```python
from build123d import *

# Parameters (mm, degrees)
F1_DEPTH  = 31.5
F2_R      = 3
F2_R_2    = 1.5
F3_DEPTH  = 5
F4_DEPTH  = 2
F2_R_3    = 4
F5_DEPTH  = 1
F6_DEPTH  = 4
F7_R      = 1.5
F8_DEPTH  = 31.5010001
F7_R_2    = 4
F9_DEPTH  = 2
F10_DEPTH = 33.501


with BuildPart() as f1:
    # F0 (on Top) → F1 (new body)
    with BuildSketch(Plane.XY):
        with BuildLine():
            Line((7.9372539332, -14.75), (0, -14.75))
            Line((0, -14.75), (0, -16.75))
            ThreePointArc((0, -16.75), (4.0926763859, -16.2423058708), (7.9372539332, -14.75))
        make_face()
        with BuildLine():
            ThreePointArc((16.75, 0), (16.2423058708, -4.0926763859), (14.75, -7.9372539332))
            Line((14.75, -7.9372539332), (14.75, -14.75))
            Line((14.75, -14.75), (7.9372539332, -14.75))
            ThreePointArc((7.9372539332, -14.75), (4.0926763859, -16.2423058708), (0, -16.75))
            Line((0, -16.75), (16.75, -16.75))
            Line((16.75, -16.75), (16.75, 0))
        make_face()
        with BuildLine():
            Line((14.75, -14.75), (14.75, -7.9372539332))
            ThreePointArc((14.75, -7.9372539332), (11.8440385849, -11.8440385849), (7.9372539332, -14.75))
            Line((7.9372539332, -14.75), (14.75, -14.75))
        make_face()
        with BuildLine():
            Line((14.75, -7.9372539332), (14.75, 0))
            ThreePointArc((14.75, 0), (10.4298250225, -10.4298250225), (0, -14.75))
            Line((0, -14.75), (7.9372539332, -14.75))
            ThreePointArc((7.9372539332, -14.75), (11.8440385849, -11.8440385849), (14.75, -7.9372539332))
        make_face()
        with BuildLine():
            ThreePointArc((0, -14.75), (10.4298250225, -10.4298250225), (14.75, 0))
            ThreePointArc((14.75, 0), (10.4298250225, 10.4298250225), (0, 14.75))
            Line((0, 14.75), (0, 12.75))
            ThreePointArc((0, 12.75), (9.0156114601, 9.0156114601), (12.75, 0))
            ThreePointArc((12.75, 0), (9.0156114601, -9.0156114601), (0, -12.75))
            Line((0, -12.75), (0, -14.75))
        make_face()
        with BuildLine():
            Line((14.75, 7.9372539332), (14.75, 0))
            Line((14.75, 0), (14.75, -7.9372539332))
            ThreePointArc((14.75, -7.9372539332), (16.2423058708, -4.0926763859), (16.75, 0))
            ThreePointArc((16.75, 0), (16.2423058708, 4.0926763859), (14.75, 7.9372539332))
        make_face()
        with BuildLine():
            ThreePointArc((0, 14.75), (10.4298250225, 10.4298250225), (14.75, 0))
            Line((14.75, 0), (14.75, 7.9372539332))
            ThreePointArc((14.75, 7.9372539332), (11.8440385849, 11.8440385849), (7.9372539332, 14.75))
            Line((7.9372539332, 14.75), (0, 14.75))
        make_face()
        with BuildLine():
            Line((14.75, 14.75), (14.75, 7.9372539332))
            ThreePointArc((14.75, 7.9372539332), (16.2423058708, 4.0926763859), (16.75, 0))
            Line((16.75, 0), (16.75, 16.75))
            Line((16.75, 16.75), (0, 16.75))
            ThreePointArc((0, 16.75), (4.0926763859, 16.2423058708), (7.9372539332, 14.75))
            Line((7.9372539332, 14.75), (14.75, 14.75))
        make_face()
        with BuildLine():
            ThreePointArc((7.9372539332, 14.75), (11.8440385849, 11.8440385849), (14.75, 7.9372539332))
            Line((14.75, 7.9372539332), (14.75, 14.75))
            Line((14.75, 14.75), (7.9372539332, 14.75))
        make_face()
        with BuildLine():
            Line((0, 16.75), (0, 14.75))
            Line((0, 14.75), (7.9372539332, 14.75))
            ThreePointArc((7.9372539332, 14.75), (4.0926763859, 16.2423058708), (0, 16.75))
        make_face()
        with BuildLine():
            Line((0, 12.75), (0, 14.75))
            ThreePointArc((0, 14.75), (-10.4298250296, 10.4298250154), (-14.75, -2e-08))
            ThreePointArc((-14.75, -2e-08), (-10.4298250154, -10.4298250296), (0, -14.75))
            Line((0, -14.75), (0, -12.75))
            ThreePointArc((0, -12.75), (-12.75, 0), (0, 12.75))
        make_face()
        with BuildLine():
            ThreePointArc((-14.75, -2e-08), (-10.4298250296, 10.4298250154), (0, 14.75))
            Line((0, 14.75), (-7.9372539332, 14.75))
            ThreePointArc((-7.9372539332, 14.75), (-11.8440385849, 11.8440385849), (-14.75, 7.9372539332))
            Line((-14.75, 7.9372539332), (-14.75, -2e-08))
        make_face()
        with BuildLine():
            Line((-7.9372539332, 14.75), (0, 14.75))
            Line((0, 14.75), (0, 16.75))
            ThreePointArc((0, 16.75), (-4.0926763859, 16.2423058708), (-7.9372539332, 14.75))
        make_face()
        with BuildLine():
            Line((-14.75, -7.9372539332), (-14.75, -2e-08))
            Line((-14.75, -2e-08), (-14.75, 7.9372539332))
            ThreePointArc((-14.75, 7.9372539332), (-16.2423058693, 4.092676392), (-16.75, 1.25e-08))
            ThreePointArc((-16.75, 1.25e-08), (-16.2423058723, -4.0926763799), (-14.75, -7.9372539332))
        make_face()
        with BuildLine():
            Line((-7.9372539332, -14.75), (0, -14.75))
            ThreePointArc((0, -14.75), (-10.4298250154, -10.4298250296), (-14.75, -2e-08))
            Line((-14.75, -2e-08), (-14.75, -7.9372539332))
            ThreePointArc((-14.75, -7.9372539332), (-11.8440385849, -11.8440385849), (-7.9372539332, -14.75))
        make_face()
        with BuildLine():
            Line((0, -16.75), (0, -14.75))
            Line((0, -14.75), (-7.9372539332, -14.75))
            ThreePointArc((-7.9372539332, -14.75), (-4.0926763859, -16.2423058708), (0, -16.75))
        make_face()
    extrude(amount=F1_DEPTH)

    # F2 (on face) → F3 (cut)
    with BuildSketch(Plane.YZ.offset(16.75)):
        with Locations((0, 24)):
            Circle(F2_R)
        with Locations((0, 24)):
            Circle(F2_R_2, mode=Mode.SUBTRACT)
        with Locations((0, 7.5)):
            Circle(F2_R)
        with Locations((0, 7.5)):
            Circle(F2_R_2, mode=Mode.SUBTRACT)
        with Locations((0, 24)):
            Circle(F2_R_2)
        with Locations((0, 7.5)):
            Circle(F2_R_2)
    extrude(amount=-F3_DEPTH, mode=Mode.SUBTRACT)

    # F2 (on face) → F4 (join)
    with BuildSketch(Plane.YZ.offset(16.75)):
        with Locations((0, 24)):
            Circle(F2_R)
        with Locations((0, 24)):
            Circle(F2_R_2, mode=Mode.SUBTRACT)
        with Locations((0, 7.5)):
            Circle(F2_R)
        with Locations((0, 7.5)):
            Circle(F2_R_2, mode=Mode.SUBTRACT)
    extrude(amount=-F4_DEPTH)

    # F2 (on face) → F5 (cut)
    with BuildSketch(Plane.YZ.offset(16.75)):
        with Locations((0, 15.75)):
            Circle(F2_R_3)
    extrude(amount=-F5_DEPTH, mode=Mode.SUBTRACT)

    # F0 (on Top) → F6 (join)
    with BuildSketch(Plane.XY):
        with BuildLine():
            ThreePointArc((12.75, 0), (9.0156114601, 9.0156114601), (0, 12.75))
            Line((0, 12.75), (0, -12.75))
            ThreePointArc((0, -12.75), (9.0156114601, -9.0156114601), (12.75, 0))
        make_face()
        with BuildLine():
            Line((0, -12.75), (0, 12.75))
            ThreePointArc((0, 12.75), (-12.75, 0), (0, -12.75))
        make_face()
    extrude(amount=F6_DEPTH)

    # F7 (on face) → F8 (cut, through all)
    with BuildSketch(Plane(origin=(0, 0, 0), x_dir=(1, 0, 0), z_dir=(0, 0, -1))):
        Circle(F7_R)
    extrude(amount=-F8_DEPTH, mode=Mode.SUBTRACT)

    # F7 (on face) → F9 (cut)
    with BuildSketch(Plane(origin=(0, 0, 0), x_dir=(1, 0, 0), z_dir=(0, 0, -1))):
        Circle(F7_R_2)
        Circle(F7_R, mode=Mode.SUBTRACT)
    extrude(amount=-F9_DEPTH, mode=Mode.SUBTRACT)

    # F2 (on face) → F10 (cut, through all)
    with BuildSketch(Plane.YZ.offset(16.75)):
        with Locations((0, 24)):
            Circle(F2_R_2)
        with Locations((0, 7.5)):
            Circle(F2_R_2)
    extrude(amount=-F10_DEPTH, mode=Mode.SUBTRACT)


solid = f1.part
```
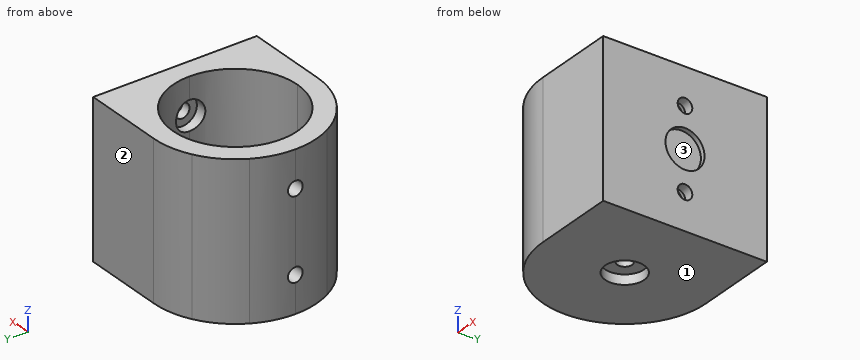
Model file for the job. Use its own axes, mm. Face numbers are marked on the shaded views. Coordinates: 2 decimals unless noted, no trailing zeros. Write each loop counter-clockwise with the first axis right and the second up, starting at its lowest first coordinate (ties: lowest second). Pieces come first, ordered by that corner, then holes. Notation, with made-up numbers: (55, 26) - (109, 26) arc R11 ccw to (109, 42) - close; hole circle Ø5 at (-4, 55). An arc over 180 degrees is marked (long way). Use a Markdown table: item, result. Add a question column.
Item 1: Band-saw the part on D-D, the plane y = 4.5. Write the cut outline in (x, z).
Item 2: Band-saw the part on C-C, the plane z = 7.5. Write the cut outline in (x, y).
Item 3: Drop flat-ended pins along their axis: pin 1 (1 mm diameter, centred on x = -3.5, y = -1.5, fed in from +Z); pin 2 (10 mm diameter, centred on y = -6.5, z = 9.5, fed in from -X); pin 3 (10 mm diameter, centred on y = 7, z = 7.5, fed in from -X). Give the stop position or say it passes through.
Item 4: Two-plate mould, pull along Z, no slides. Class the marked faces 1, 2 and 3: pulls with the +Z half, pulls with the -Z half, needs draft (parallel to the pull), parting line crosses it, or undercut.
Item 5: Drill centre lines: line 1 along Z through (x, y) = (-15.6, 0); line 2 along Z through (x, y) = (16.1, 0); line 3 along Y through (x, z) = (0.5, 8.5). Where is each one in solid material? Low to high.
Item 6: Band-saw the part on B-B, the plane x = -0.5. Write the cut outline in (y, z), and give its area (3 significant figures).
Item 7: Band-saw the part on A-A, the plane z = 15.75. Write the cut outline in (x, y).
A:
| question | item | result |
|---|---|---|
| 1 | outline | (-16.13, 0) - (16.75, 0) - (16.75, 31.5) - (11.93, 31.5) - (11.93, 4) - (-11.93, 4) - (-11.93, 31.5) - (-16.13, 31.5) - close |
| 2 | outline | (-16.68, -1.5) arc R16.75 ccw to (0, -16.75) - (16.75, -16.75) - (16.75, -1.5) - (14.75, -1.5) - (14.75, -3) - (12.39, -3) arc R12.75 cw to (-12.66, -1.5) - close; (-16.68, 1.5) - (-12.66, 1.5) arc R12.75 cw to (12.39, 3) - (14.75, 3) - (14.75, 1.5) - (16.75, 1.5) - (16.75, 16.75) - (0, 16.75) arc R16.75 ccw to start |
| 3 | pin 1 | stops at z = 4 |
| 3 | pin 2 | stops at x = -16.68 |
| 3 | pin 3 | stops at x = -16.63 |
| 4 | face 1 | pulls with the -Z half |
| 4 | face 2 | needs draft |
| 4 | face 3 | undercut |
| 5 | line 1 | z = 0 to 6, 9 to 22.5, 25.5 to 31.5 |
| 5 | line 2 | z = 0 to 6, 9 to 11.75, 19.75 to 22.5, 25.5 to 31.5 |
| 5 | line 3 | y = -16.75 to -12.74, 12.74 to 16.75 |
| 6 | outline | (-16.74, 0) - (-3.97, 0) - (-3.97, 2) - (-1.41, 2) - (-1.41, 4) - (-12.74, 4) - (-12.74, 31.5) - (-16.74, 31.5) - close; (1.41, 2) - (3.97, 2) - (3.97, 0) - (16.74, 0) - (16.74, 31.5) - (12.74, 31.5) - (12.74, 4) - (1.41, 4) - close |
| 6 | area | 333 mm² |
| 7 | outline | (0, -16.75) - (16.75, -16.75) - (16.75, -4) - (15.75, -4) - (15.75, 4) - (16.75, 4) - (16.75, 16.75) - (0, 16.75) arc R16.75 ccw to start; hole circle Ø25.5 at (0, 0) |
